```python
from build123d import *

# Parameters (mm, degrees)
SKETCH1_R                                    = 23
BOSS_EXTRUDE1_DEPTH                          = 17
SHELL1_T                                     = -2.6
SKETCH4_R                                    = 4.5
BOSS_EXTRUDE3_DEPTH                          = 5
SKETCH5_R                                    = 3.325
CUT_EXTRUDE2_DEPTH                           = 34.857938508
SKETCH22_R                                   = 20.4
SKETCH22_R_2                                 = 17.6
BOSS_EXTRUDE10_DEPTH                         = 14.4
SKETCH24_R                                   = 2.5
BOSS_EXTRUDE11_DEPTH                         = 6.8
CSK_SLOT_FOR_M1_6_COUNTERSUNK_FLAT_H_2_COUNT = 2
CSK_SLOT_FOR_M1_6_COUNTERSUNK_FLAT_H_2_PITCH = 27.712812921
CSK_SLOT_FOR_M1_6_COUNTERSUNK_FLAT_H_3_COUNT = 2
CSK_SLOT_FOR_M1_6_COUNTERSUNK_FLAT_H_3_PITCH = 27.712812921
BOSS_EXTRUDE12_DEPTH                         = 6
SKETCH29_W                                   = 2
SKETCH29_H                                   = 3
CUT_EXTRUDE5_DEPTH                           = 47.005728796
FILLET2_R                                    = 2
SKETCH30_W                                   = 8
SKETCH30_H                                   = 3.3
CUT_EXTRUDE6_DEPTH                           = 4.5
BOSS_EXTRUDE13_DEPTH                         = 0.6
BOSS_EXTRUDE14_DEPTH                         = 0.6
CUT_EXTRUDE7_START                           = -13.6
CUT_EXTRUDE7_DEPTH                           = 13.6


# Read off the part's stored shape, not the designer's step: Cut-Extrude7
with BuildPart() as part:
    # Sketch1 → Boss-Extrude1 (new body)
    with BuildSketch(Plane(origin=(0, 0, 0), x_dir=(1, 0, 0), z_dir=(0, 1, 0))):
        with Locations(Location((0, 0, 0), (0, 0, 270))):
            Circle(SKETCH1_R)
    extrude(amount=BOSS_EXTRUDE1_DEPTH)

    # Shell1
    shell1_openings = [part.faces().sort_by_distance(p)[0] for p in [
        (0, 17, 0),
    ]]
    offset(amount=SHELL1_T, openings=shell1_openings, kind=Kind.INTERSECTION)

    # Sketch4 → Boss-Extrude3 (add)
    with BuildSketch(Plane(origin=(0, 2.6, 0), x_dir=(1, 0, 0), z_dir=(0, 1, 0))):
        with Locations(Location((0, 0, 0), (0, 0, 270))):
            Circle(SKETCH4_R)
    extrude(amount=BOSS_EXTRUDE3_DEPTH)

    # Sketch5 → Cut-Extrude2 (cut, through all)
    with BuildSketch(Plane(origin=(0, 7.6, 0), x_dir=(1, 0, 0), z_dir=(0, 1, 0))):
        with Locations(Location((0, 0, 0), (0, 0, 270))):
            Circle(SKETCH5_R)
    extrude(amount=-CUT_EXTRUDE2_DEPTH, mode=Mode.SUBTRACT)

    # Sketch22 → Boss-Extrude10 (add)
    with BuildSketch(Plane(origin=(0, 2.6, 0), x_dir=(1, 0, 0), z_dir=(0, 1, 0))):
        Circle(SKETCH22_R)
        with Locations(Location((0, 0, 0), (0, 0, 270))):
            Circle(SKETCH22_R_2, mode=Mode.SUBTRACT)
    extrude(amount=BOSS_EXTRUDE10_DEPTH)

    # Sketch24 → Boss-Extrude11 (add)
    with BuildSketch(Plane(origin=(0, 2.6, 0), x_dir=(1, 0, 0), z_dir=(0, 1, 0))):
        with Locations((-8, 13.856406461)):
            Circle(SKETCH24_R)
        with Locations((16, 0)):
            Circle(SKETCH24_R)
        with Locations((-8, -13.856406461)):
            Circle(SKETCH24_R)
    extrude(amount=BOSS_EXTRUDE11_DEPTH)

    # Sketch26 → CSK SLOT for M1.6 Countersunk Flat Head (revolve, cut)
    with BuildSketch(Plane(origin=(-8, 0, 13.856406461), x_dir=(0, 0, -1), z_dir=(1, 0, 0))):
        Polygon((0, 0), (0, 17), (0.9, 17), (0.9, 8.4), (1.8, 7.5), (1.8, 0), align=None)
    csk_slot_for_m1_6_countersunk_flat_head = revolve(axis=Axis((-8, -6.35, 13.856406461), (0, 1, 0)), mode=Mode.SUBTRACT)

    # CSK SLOT for M1.6 Countersunk Flat H 2: CSK SLOT for M1.6 Countersunk Flat Head ×2
    with Locations(*[(0, 0, -i * CSK_SLOT_FOR_M1_6_COUNTERSUNK_FLAT_H_2_PITCH) for i in range(1, CSK_SLOT_FOR_M1_6_COUNTERSUNK_FLAT_H_2_COUNT)]):
        add(csk_slot_for_m1_6_countersunk_flat_head, mode=Mode.SUBTRACT)

    # CSK SLOT for M1.6 Countersunk Flat H 3: CSK SLOT for M1.6 Countersunk Flat Head ×2
    with Locations(*[Vector(0.8660254037844364, 0, -0.5000000000000041) * (i * CSK_SLOT_FOR_M1_6_COUNTERSUNK_FLAT_H_3_PITCH) for i in range(1, CSK_SLOT_FOR_M1_6_COUNTERSUNK_FLAT_H_3_COUNT)]):
        add(csk_slot_for_m1_6_countersunk_flat_head, mode=Mode.SUBTRACT)

    # Sketch28 → Boss-Extrude12 (add)
    with BuildSketch(Plane.XZ):
        with BuildLine():
            Line((-1.694333823, 2.860919065), (-5.263926338, 9.085385824))
            Line((-5.263926338, 9.085385824), (-10.902522986, 5.851776718))
            Line((-10.902522986, 5.851776718), (2.031913438, -16.702609871))
            Line((2.031913438, -16.702609871), (7.670510085, -13.469000765))
            Line((7.670510085, -13.469000765), (1.613572817, -2.907233696))
            ThreePointArc((1.613572817, -2.907233696), (-2.884359054, -1.654115427), (-1.694333823, 2.860919065))
        make_face()
        with BuildLine():
            Line((0.374670309, 12.31899493), (-5.263926338, 9.085385824))
            Line((-5.263926338, 9.085385824), (-1.694333823, 2.860919065))
            ThreePointArc((-1.694333823, 2.860919065), (1.646506155, 2.888709484), (3.325, 0))
            ThreePointArc((3.325, 0), (2.865375597, -1.686786202), (1.613572817, -2.907233696))
            Line((1.613572817, -2.907233696), (7.670510085, -13.469000765))
            Line((7.670510085, -13.469000765), (13.309106732, -10.23539166))
            Line((13.309106732, -10.23539166), (0.374670309, 12.31899493))
        make_face()
    extrude(amount=BOSS_EXTRUDE12_DEPTH)

    # Sketch29 → Cut-Extrude5 (cut, through all)
    with BuildSketch(Plane(origin=(-5.223545836, 0, 9.108543139), x_dir=(0.8674764072728275, 0, 0.4974783239750529), z_dir=(-0.4974783239750529, 0, 0.8674764072728275))):
        with Locations((-5.546549396, -1.5)):
            Rectangle(SKETCH29_W, SKETCH29_H)
        with Locations((5.453450604, -1.5)):
            Rectangle(SKETCH29_W, SKETCH29_H)
    extrude(amount=-CUT_EXTRUDE5_DEPTH, mode=Mode.SUBTRACT)

    # Fillet2
    fillet2_edges = [part.edges().sort_by_distance(p)[0] for p in [
        (-10.902522986, -4.5, 5.851776718),
        (0.374670309, -4.5, 12.31899493),
        (-5.263926338, -6, 9.085385824),
    ]]
    fillet(fillet2_edges, radius=FILLET2_R)

    # Sketch30 → Cut-Extrude6 (cut)
    with BuildSketch(Plane(origin=(-5.223545836, 0, 9.108543139), x_dir=(0.8674764072728275, 0, 0.4974783239750529), z_dir=(-0.4974783239750529, 0, 0.8674764072728275))):
        with Locations((-0.046549396, -4.35)):
            Rectangle(SKETCH30_W, SKETCH30_H)
    extrude(amount=-CUT_EXTRUDE6_DEPTH, mode=Mode.SUBTRACT)

    # Sketch31 → Boss-Extrude13 (add)
    with BuildSketch(Plane.XZ.offset(6)):
        Polygon((-6.49517951, 3.191828695), (0.444631749, 7.171655287), (-1.147298888, 9.94757979), (-8.087110146, 5.967753198), align=None)
    extrude(amount=-BOSS_EXTRUDE13_DEPTH)

    # Sketch33 → Boss-Extrude14 (add)
    with BuildSketch(Plane(origin=(0, -5.4, 0), x_dir=(1, 0, 0), z_dir=(0, 1, 0))):
        Polygon((-6.49517951, -3.191828695), (0.444631749, -7.171655287), (-0.550324899, -8.906608101), (-7.490136157, -4.92678151), align=None)
    extrude(amount=BOSS_EXTRUDE14_DEPTH)

    # Cut-Extrude7 outline → Cut-Extrude7 (cut)
    with BuildSketch(Plane.XZ.offset(6).offset(CUT_EXTRUDE7_START)):
        with BuildLine():
            Line((-3.118548226, 1.324113199), (-3.026514963, 1.376892218))
            ThreePointArc((-3.026514963, 1.376892218), (-1.654115427, 2.884359054), (0.340085146, 3.307562107))
            Line((0.340085146, 3.307562107), (0.351357403, 3.314026495))
            Line((0.351357403, 3.314026495), (-2.882251703, 8.952623142))
            Line((-2.882251703, 8.952623142), (-6.352157332, 6.962709846))
            Line((-6.352157332, 6.962709846), (-3.118548226, 1.324113199))
        make_face()
    extrude(amount=CUT_EXTRUDE7_DEPTH, mode=Mode.SUBTRACT)


solid = part.part
```
Check sheet for the modelled part. Datum: model origin and axes. Units: mm. A direction names the side the tool comes from. Round coordinates to 2 decimals unless told otherwise and drop trailing zeros. Order: outer loops, then holes, each group sorted by start corner. A loop starts at its lowest first (then second) coordinate and runs counter-clockwise, first axis right, second up. Notation, with made-up numbers: M 10,-11 L 30,-11 A6 cw 30,-6 Z; hole C -5.5,-1 d8. An arc over 180 degrees is marked long. Answer in a Markdown table with one row per item.
(1) Material ranges on line 1 along X through (y, z) = (7.5, 0) (3 decimals); line 2 along X through (y, z) = (8.7, 0); line 3 along Y through (x, z) = (11.5, -9), recorded low to high. Write a range as from..to.
Findings:
| item | result |
|---|---|
| line 1 | x = -23..-17.6, -4.5..-3.325, 3.325..4.5, 13.5..14.2, 17.8..23 |
| line 2 | x = -23..-17.6, 13.5..15.1, 16.9..23 |
| line 3 | y = -6..-3, 0..2.6 |
(2) Gauge pin test, flat ends, axial feed: pin 1 (12 mm diameter, centred on y = 4.5, z = 11.5, fed in from -X); pin 2 (6.5 mm diameter, centred on x = -4, z = 7.5, fed in from -Y); pin 3 (3 mm diameter, centred on x = -8, z = -13.86, fed in from -Y); pin 4 (4 mm diameter, centred on x = -14.5, y = 3.5, fed in from +Z). Record the tip position at first contact, or that the pin passes through.
Findings:
| item | result |
|---|---|
| pin 1 | stops at x = -22.33 |
| pin 2 | stops at y = -6 |
| pin 3 | stops at y = 7.8 |
| pin 4 | stops at z = 19.31 |
(3) Section check A-A on y = 1.5. Record the boundary of the cut face in (x, z) (3 decimals).
Findings:
| item | result |
|---|---|
| outline | C 0,0 d46; hole C -8,-13.856 d3.6; hole C -8,13.856 d3.6; hole M -6.352,6.963 L -3.119,1.324 L -3.027,1.377 A3.325 ccw long 0.34,3.308 L 0.351,3.314 L -2.882,8.953 Z; hole C 16,0 d3.6 |
(4) Set-up check for faces 4 (the flat face through (-4, -3, -5)), 5 (the cylindrical face through (-6.4, 3.7, 13.03)), 6 (the flat face through (-7, -5.4, 6)), 7 (the flat face through (-4.02, -4.48, -6.15)): record each of +Z, -Z, +X, -X, +Y, -Y from which the full face is reachable in a straight line by a thin tool's end or side.
Findings:
| item | result |
|---|---|
| face 4 | -Z, -X |
| face 5 | -Y |
| face 6 | +Z |
| face 7 | -Z, -X, -Y |
(5) Draft check along Y on faces 1 (the flat face through (-4.4, -0.62, 3.56)), 2 (the flat face through (-5.64, -3.74, 3.68)), 3 (the flat face through (4, -6, -3)). Enter one of: +Y half, -Y half, draft (parallel to the pull), parting line (faces both ways), or undercut.
Findings:
| item | result |
|---|---|
| face 1 | draft |
| face 2 | undercut |
| face 3 | -Y half |
(6) Section check B-B on z = -6.5. Record the boundary of the cut face in (x, y).
Findings:
| item | result |
|---|---|
| outline | M -22.06,0 L -1.51,0 L -1.51,-3 L -3.82,-3 L -3.82,-6 L 11.17,-6 L 11.17,-3 L 8.86,-3 L 8.86,0 L 22.06,0 L 22.06,17 L 16.36,17 L 16.36,2.6 L -16.36,2.6 L -16.36,17 L -22.06,17 Z |
